Source: CAD feature listing. Evaluate the final solid. Frame: model axes, mm. Face numbers are marked on the shaded views. Give positions to 0.01 mm unless a question says otherwise; leave off trailing zeros. Write each loop counter-clockwise with the first axis right and the second up, starting at its lowest first coordinate (ties: lowest second). Pieces come first, ordered by that corner, then holes. Notation, with made-up numbers: (20.25, 89) -> (62.25, 89) arc R18 cw to (62.25, 95) -> close; hole circle Ø4 at (-7.5, -3). An arc over 180 degrees is marked (long way). Use a Markdown table: item, result. Add a question column.
Autodesk Inventor part; units mm, degrees
ref_plane "YZ Plane" through (0, 0, 0) normal (1, 0, 0) x (0, 1, 0)
ref_plane "XZ Plane" through (0, 0, 0) normal (0, 1, 0) x (-1, 0, 0)
ref_plane "XY Plane" through (0, 0, 0) normal (0, 0, 1) x (1, 0, 0)
ref_plane "Work Plane1" through (0, 0, 0) normal (0, 0, 1) x (1, 0, 0)
sketch "Sketch1" plane through (0, 0, 0) normal (0, 0, 1) x (1, 0, 0)
  line L0 (45, 45) -> (-45, 45)
  line L1 (-45, 45) -> (-45, -45)
  line L2 (-45, -45) -> (45, -45)
  line L3 (45, -45) -> (45, 45)
  line L4 (45, 45) -> (-45, -45) construction
  line L5 (-45, 45) -> (45, -45) construction
  circle A0 centre (19, 19) radius 2.4585
  circle A1 centre (19, -19) radius 2.4585
  circle A2 centre (-19, -19) radius 2.4585
  circle A3 centre (-19, 19) radius 2.4585
  point P0 (0, 0)
  point P1 (0, 0)
  dimension "d0" = 90
  dimension "d1" = 90
extrude "Extrusion1" add sketch "Sketch1" along normal blind 10
properties part number "Sujeción Cilindro Cortadora"
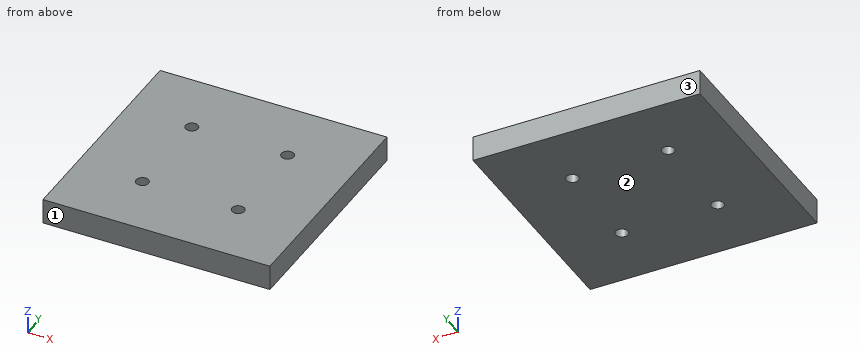
(1) Cut plane A-A on y = -19. Return the cut outline in (x, z), then the cut area to 3 significant figures.
(2) Material intervals for L1, parallel to Y at x = 19, z = 6.25; L2, parallel to X at y = -19.5, z = 1.25, sorted ascending.
(3) Mould query, pull axis Y, two halves, no side actions, for the marked faces 1, 2 and 3. Classes: +Y half, -Y half, draft (parallel to the pull), parting line (faces both ways), or undercut.
Output:
| question | item | result |
|---|---|---|
| 1 | outline | (-45, 0) -> (-21.46, 0) -> (-21.46, 10) -> (-45, 10) -> close; (-16.54, 0) -> (16.54, 0) -> (16.54, 10) -> (-16.54, 10) -> close; (21.46, 0) -> (45, 0) -> (45, 10) -> (21.46, 10) -> close |
| 1 | area | 802 mm^2 |
| 2 | L1 | -45 to -21.46, -16.54 to 16.54, 21.46 to 45 |
| 2 | L2 | -45 to -21.41, -16.59 to 16.59, 21.41 to 45 |
| 3 | face 1 | -Y half |
| 3 | face 2 | draft |
| 3 | face 3 | +Y half |
